The model under review builds one solid part; all positions refer to its coordinate system, in mm. A direction names the side the tool comes from. Coordinates: 2 decimals unless noted, no trailing zeros. Loops run counter-clockwise (first coordinate to the right, second up) from the corner with the lowest first, then second, coordinate; pieces in that order, holes last. Notation, with made-up numbers: (-9, -39.5) - (31, -39.5) arc R16 ccw to (31, -12.5) - close; hole circle Ø10 at (15.25, -39.75). An arc over 180 degrees is marked (long way). Use a Markdown table: item, result. Add a question column.
1) Add section A-A, the plane z = 62.07. Give the boundary of the cut face in (x, y) (3 decimals).
2) To check wall thickness, follow L1, parallel to X at y = -20.69, z = -0.75 (3 decimals); L2, parallel to Y at x = 0, z = -1 (3 decimals); L3, parallel to Z at x = 0, y = 42.6 (3 decimals). State the ranges of each line that lie inside material, in increasing order. Write a range as [from, to].
3) Add section B-B, the plane y = -20.69. Give the boundary of the cut face in (x, z) (3 decimals), and give its area (3 significant figures).
4) The part is to be moulded in two halves that separate along Z. For faces 1 (the cylindrical face through (-0.33, 42.65, 59.59)), 2 (the flat face through (0, 0, -2)), 3 (the cylindrical face through (-0.325, 42.653, 30.556)), 4 (the cylindrical face through (-0.325, 10.824, -0.727)), say which applies: pulls with the +Z half, pulls with the -Z half, needs draft (parallel to the pull), parting line crosses it, or undercut.
5) For faces 5 (the flat face through (0, 0, 0)), 6 (the cylindrical face through (1.15, -22.91, -0.73)), list the 3-axis set-ups (+Z, -Z, +X, -X, +Y, -Y) from which the entire face can be reached by the end or side of a thin tool; tool diameter is ignored.
6) Add section D-D, the plane x = 12. Give the boundary of the cut face in (y, z).
7) Clearance check with flat-ended pins moving along their axes: pin 1 (8 mm diameter, centred on x = 0, z = 62.07, fed in from -Y); pin 2 (6 mm diameter, centred on x = 0, y = -20.69, fed in from +Z). State where each tip first meets the part, or that it passes through.
8) Add section C-C, the plane x = 0. Give the number of separate pieces and of enclosed holes in the cut face, and give its area (3 significant figures).
```python
from build123d import *

# Parameters (mm, degrees)
SKETCH1_W                       = 37.75
SKETCH1_H                       = 82.76
BASE_FLANGE1_DEPTH              = 2
EDGE_FLANGE1_STRIP_W            = 12
EDGE_FLANGE1_STRIP_H            = 2
EDGE_FLANGE1_STRIP_CUT_DEPTH    = 37.75
EDGE_FLANGE1_DEPTH              = 37.75
M6X1_0_TAPPED_HOLE2_D           = 5
M6X1_0_TAPPED_HOLE2_DEPTH       = 15
M6X1_0_TAPPED_HOLE2_CSINK_D     = 6.05
M6X1_0_TAPPED_HOLE2_CSINK_ANGLE = 90
M6X1_0_TAPPED_HOLE2_TIP         = 1.502151548
M6X1_0_TAPPED_HOLE3_D           = 5
M6X1_0_TAPPED_HOLE3_DEPTH       = 15
M6X1_0_TAPPED_HOLE3_CSINK_D     = 6.05
M6X1_0_TAPPED_HOLE3_CSINK_ANGLE = 90
M6X1_0_TAPPED_HOLE3_TIP         = 1.502151548


# Sheet-metal steps are written as plain solids
with BuildPart() as part:
    # Sketch1 → Base-Flange1 (new body)
    with BuildSketch(Plane.XY):
        Rectangle(SKETCH1_W, SKETCH1_H)
    extrude(amount=-BASE_FLANGE1_DEPTH)

    # Edge-Flange1 strip (across the edge) → Edge-Flange1 strip cut (cut)
    with BuildSketch(Plane(origin=(18.875, 41.38, 0), x_dir=(0, -1, 0), z_dir=(-1, 0, 0))):
        with Locations((-4, -1)):
            Rectangle(EDGE_FLANGE1_STRIP_W, EDGE_FLANGE1_STRIP_H)
    extrude(amount=EDGE_FLANGE1_STRIP_CUT_DEPTH, mode=Mode.SUBTRACT)

    # Edge-Flange1 section (across the edge) → Edge-Flange1 (add)
    with BuildSketch(Plane(origin=(18.875, 41.38, 0), x_dir=(0, -1, 0), z_dir=(-1, 0, 0))):
        with BuildLine():
            Line((-2, 2), (-2, 82.76))
            Line((-2, 82.76), (0, 82.76))
            Line((0, 82.76), (0, 2))
            ThreePointArc((0, 2), (0.585786438, 0.585786438), (2, 0))
            Line((2, 0), (2, -2))
            ThreePointArc((2, -2), (-0.828427125, -0.828427125), (-2, 2))
        make_face()
    extrude(amount=EDGE_FLANGE1_DEPTH)

    # M6x1.0 Tapped Hole2
    with Locations(Plane(origin=(0, 0, -2), x_dir=(-1, 0, 0), z_dir=(0, 0, -1))):
        with Locations((0, 8.345), (0, -20.69)):
            CounterSinkHole(M6X1_0_TAPPED_HOLE2_D / 2, M6X1_0_TAPPED_HOLE2_CSINK_D / 2, depth=M6X1_0_TAPPED_HOLE2_DEPTH, counter_sink_angle=M6X1_0_TAPPED_HOLE2_CSINK_ANGLE)
            with Locations((0, 0, -(M6X1_0_TAPPED_HOLE2_DEPTH + M6X1_0_TAPPED_HOLE2_TIP / 2))):  # 118° drill point
                Cone(0, M6X1_0_TAPPED_HOLE2_D / 2, M6X1_0_TAPPED_HOLE2_TIP, mode=Mode.SUBTRACT)

    # M6x1.0 Tapped Hole3
    with Locations(Plane(origin=(0, 41.38, 0), x_dir=(-1, 0, 0), z_dir=(0, -1, 0))):
        with Locations((0, -33.035), (0, -62.07)):
            CounterSinkHole(M6X1_0_TAPPED_HOLE3_D / 2, M6X1_0_TAPPED_HOLE3_CSINK_D / 2, depth=M6X1_0_TAPPED_HOLE3_DEPTH, counter_sink_angle=M6X1_0_TAPPED_HOLE3_CSINK_ANGLE)
            with Locations((0, 0, -(M6X1_0_TAPPED_HOLE3_DEPTH + M6X1_0_TAPPED_HOLE3_TIP / 2))):  # 118° drill point
                Cone(0, M6X1_0_TAPPED_HOLE3_D / 2, M6X1_0_TAPPED_HOLE3_TIP, mode=Mode.SUBTRACT)


solid = part.part
```
From the geometry:
| question | item | result |
|---|---|---|
| 1 | outline | (-18.875, 41.38) - (-3.025, 41.38) - (-2.5, 41.905) - (-2.5, 43.38) - (-18.875, 43.38) - close; (2.5, 41.905) - (3.025, 41.38) - (18.875, 41.38) - (18.875, 43.38) - (2.5, 43.38) - close |
| 2 | L1 | x = [-18.875, -2.5], [2.5, 18.875] |
| 2 | L2 | y = [-41.38, -23.19], [-18.19, 5.845], [10.845, 42.026] |
| 2 | L3 | z = [-0.373, 30.535], [35.535, 59.57], [64.57, 82.76] |
| 3 | outline | (-18.875, -2) - (-3.025, -2) - (-2.5, -1.475) - (-2.5, 0) - (-18.875, 0) - close; (2.5, -1.475) - (3.025, -2) - (18.875, -2) - (18.875, 0) - (2.5, 0) - close |
| 3 | area | 65.2 mm^2 |
| 4 | face 1 | undercut |
| 4 | face 2 | pulls with the -Z half |
| 4 | face 3 | undercut |
| 4 | face 4 | needs draft |
| 5 | face 5 | +Z, +X, -X, -Y |
| 5 | face 6 | +Z, -Z |
| 6 | outline | (-41.38, -2) - (39.38, -2) arc R4 ccw to (43.38, 2) - (43.38, 82.76) - (41.38, 82.76) - (41.38, 2) arc R2 cw to (39.38, 0) - (-41.38, 0) - close |
| 7 | pin 1 | stops at y = 41.38 |
| 7 | pin 2 | stops at z = 0 |
| 8 | separate pieces | 5 |
| 8 | enclosed holes | 0 |
| 8 | area | 291 mm^2 |
